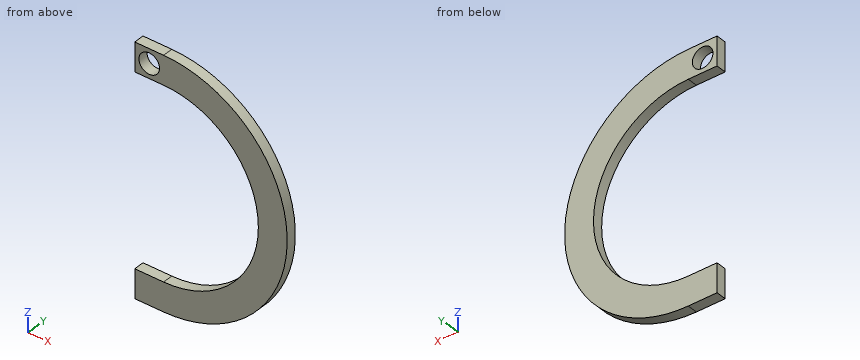
from build123d import *

# Parameters (mm, degrees)
F0_W     = 8.89
F0_H     = 8.89
F0_R     = 3.175
F1_DEPTH = 3.175


with BuildPart() as f1:
    # F0 (on Front) → F1 (new body)
    with BuildSketch(Plane.XZ):
        with Locations((0, 33.655)):
            Rectangle(F0_W, F0_H)
        with Locations((0, 33.655)):
            Circle(F0_R, mode=Mode.SUBTRACT)
        with Locations((0, -33.655)):
            Rectangle(F0_W, F0_H)
        with BuildLine():
            ThreePointArc((4.445, -38.1), (42.545, 0), (4.445, 38.1))
            Line((4.445, 38.1), (4.445, 29.21))
            ThreePointArc((4.445, 29.21), (33.655, 0), (4.445, -29.21))
            Line((4.445, -29.21), (4.445, -38.1))
        make_face()
    extrude(amount=F1_DEPTH)


solid = f1.part
CAD build for the part. Positions are in the model's coordinates, mm. Round coordinates to 2 decimals unless told otherwise and drop trailing zeros. Write each loop counter-clockwise with the first axis right and the second up, starting at its lowest first coordinate (ties: lowest second). Pieces come first, ordered by that corner, then holes. Notation, with made-up numbers: M 52,-23.5 L 62,-23.5 A38 ccw 62,15.5 Z; hole C 9,10 d6. An arc over 180 degrees is marked long. Put each result on its own line as item: value. Start each with the question number.
1) Saw through at B-B, the plane y = -1.4. Write the cut outline in (x, z) (3 decimals).
2) Drill centre lines: probe 1 along Z at (x, y) = (0, -2.2); probe 2 along X at (y, z) = (-0.6, -0.5); probe 3 along Z at (x, y) = (17.5, -0.85). Where is each one in solid material? Low to high. Write a range as [from, to].
3) Saw through at A-A, the plane x = 0. Write the cut outline in (y, z) (3 decimals), and give its area (3 significant figures).
4) Pin check, flat tips, straight feed: pin 1 Ø1 at (y, z) = (-2, -26) entering from +X; pin 2 Ø1 at (x, y) = (19, -2) entering from +Z. Stop position of each tip, or through.
5) Saw through at C-C, the plane x = 18.5. Write the cut outline in (y, z) (3 decimals), and give its area (3 significant figures).
6) Saw through at D-D, the plane z = 0. Write the cut outline in (x, y) (3 decimals).
Resolved:
1. outline: M -4.445,-38.1 L 4.445,-38.1 A38.1 ccw 4.445,38.1 L -4.445,38.1 L -4.445,29.21 L 4.445,29.21 A29.21 cw 4.445,-29.21 L -4.445,-29.21 Z; hole C 0,33.655 d6.35
2. probe 1: [-38.1, -29.21], [29.21, 30.48], [36.83, 38.1]
2. probe 2: [33.65, 42.54]
2. probe 3: [-35.79, -26.13], [26.13, 35.79]
3. outline: M -3.175,-38.1 L 0,-38.1 L 0,-29.21 L -3.175,-29.21 Z; M -3.175,29.21 L 0,29.21 L 0,30.48 L -3.175,30.48 Z; M -3.175,36.83 L 0,36.83 L 0,38.1 L -3.175,38.1 Z
3. area: 36.3 mm²
4. pin 1: x = 32.75
4. pin 2: z = 35.41
5. outline: M -3.175,-35.413 L 0,-35.413 L 0,-25.606 L -3.175,-25.606 Z; M -3.175,25.606 L 0,25.606 L 0,35.413 L -3.175,35.413 Z
5. area: 62.3 mm²
6. outline: M 33.655,-3.175 L 42.545,-3.175 L 42.545,0 L 33.655,0 Z
